```python
from build123d import *

# Parameters (mm, degrees)
SKETCH3_R           = 4.5
BOSS_EXTRUDE1_DEPTH = 18
FILLET1_R           = 5
FILLET2_R           = 5
CUT_EXTRUDE2_DEPTH  = 19.0000001


with BuildPart() as part:
    # Sketch3 → Boss-Extrude1 (new body)
    with BuildSketch(Plane.XY):
        with BuildLine():
            Line((-31.929873349, -122.5), (31.929873349, -122.5))
            ThreePointArc((31.929873349, -122.5), (38.210043039, -120.281996444), (41.704324989, -114.611893732))
            Line((41.704324989, -114.611893732), (73.308387301, 31.660797012))
            ThreePointArc((73.308387301, 31.660797012), (0, 122.5), (-73.308387301, 31.660797012))
            Line((-73.308387301, 31.660797012), (-41.704324989, -114.611893732))
            ThreePointArc((-41.704324989, -114.611893732), (-38.210043039, -120.281996444), (-31.929873349, -122.5))
        make_face()
        with Locations((50, -12.5)):
            Circle(SKETCH3_R, mode=Mode.SUBTRACT)
        with Locations((50, 87.5)):
            Circle(SKETCH3_R, mode=Mode.SUBTRACT)
        with Locations((-50, 87.5)):
            Circle(SKETCH3_R, mode=Mode.SUBTRACT)
        with Locations((-50, -12.5)):
            Circle(SKETCH3_R, mode=Mode.SUBTRACT)
        with BuildLine():
            Line((-31.929873349, -112.5), (-51.284518999, -22.921132901))
            ThreePointArc((-51.284518999, -22.921132901), (-39.736825778, -10.282511582), (-55.472323677, -3.538768301))
            Line((-55.472323677, -3.538768301), (-63.533935661, 33.772690744))
            ThreePointArc((-63.533935661, 33.772690744), (-64.271528905, 57.204152316), (-56.648842383, 79.373322021))
            ThreePointArc((-56.648842383, 79.373322021), (-41.800877501, 80.940702001), (-43.531035666, 95.770580418))
            ThreePointArc((-43.531035666, 95.770580418), (0, 112.5), (43.531035666, 95.770580418))
            ThreePointArc((43.531035666, 95.770580418), (41.800877501, 80.940702001), (56.648842383, 79.373322021))
            ThreePointArc((56.648842383, 79.373322021), (64.271528905, 57.204152316), (63.533935661, 33.772690744))
            Line((63.533935661, 33.772690744), (55.472323677, -3.538768301))
            ThreePointArc((55.472323677, -3.538768301), (39.736825778, -10.282511582), (51.284518999, -22.921132901))
            Line((51.284518999, -22.921132901), (31.929873349, -112.5))
            Line((31.929873349, -112.5), (-31.929873349, -112.5))
        make_face(mode=Mode.SUBTRACT)
    extrude(amount=BOSS_EXTRUDE1_DEPTH)

    # Fillet1
    fillet1_edges = [part.edges().sort_by_distance(p)[0] for p in [
        (-31.929873349, -112.5, 9),
        (31.929873349, -112.5, 9),
    ]]
    fillet(fillet1_edges, radius=FILLET1_R)

    # Fillet2
    fillet2_edges = [part.edges().sort_by_distance(p)[0] for p in [
        (51.284518999, -22.921132901, 9),
        (55.472323677, -3.538768301, 9),
        (56.648842383, 79.373322021, 9),
        (43.531035666, 95.770580418, 9),
        (-43.531035666, 95.770580418, 9),
        (-56.648842383, 79.373322021, 9),
        (-55.472323677, -3.538768301, 9),
        (-51.284518999, -22.921132901, 9),
    ]]
    fillet(fillet2_edges, radius=FILLET2_R)

    # Sketch5 → Cut-Extrude2 (cut, through all)
    with BuildSketch(Plane.XY.offset(18)):
        Polygon((47.724403212, -39.39837277), (54.444339069, -31.972010438), (57.506356145, -41.47554836), (172.58444794, 157.130363262), (-148.336678287, 157.130363262), (-57.506356145, -41.47554836), (-54.443982463, -31.973660914), (-47.723687693, -39.401684395), align=None)
    extrude(amount=-CUT_EXTRUDE2_DEPTH, mode=Mode.SUBTRACT)


solid = part.part
```
The listing builds one solid part. Answer for the finished solid, in the listing's coordinates (mm). A direction names the side the tool comes from. Give positions to 0.01 mm unless a question says otherwise; leave off trailing zeros. Order: outer loops, then holes, each group sorted by start corner. A loop starts at its lowest first (then second) coordinate and runs counter-clockwise, first axis right, second up.
1) Find section D-D on y = -116.5. Write down the section's boundary in (x, z).
Reported:
outline: (-41.1, 0) - (41.1, 0) - (41.1, 18) - (-41.1, 18) - close
2) For faces 4 (the face through (40.36, -73.49, 8.87)), 5 (the face through (-38.284, -120.222, 8.874)), determine the directions among +Z, -Z, +X, -X, +Y, -Y from which every point of the face is accessible in a straight line to the end or side of a thin tool.
Reported:
face 4: +Z, -Z, +Y
face 5: +Z, -Z, -X, -Y
3) Consider line 1 along Y through (x, z) = (19, 17); line 2 along X through (y, z) = (-50, 16.75); line 3 along X through (y, z) = (-42, 8). Determine where each line is inside the solid, lowest interval first.
Reported:
line 1: y = -122.5 to -112.5
line 2: x = -55.66 to -45.43, 45.43 to 55.66
line 3: x = -57.39 to -47.16, 47.16 to 57.39
4) Find section C-C on x = 1. Write down the section's boundary in (y, z), then the cut area to 3 significant figures.
Reported:
outline: (-122.5, 0) - (-112.5, 0) - (-112.5, 18) - (-122.5, 18) - close
area: 180 mm2
5) Find section B-B on y = -51. Write down the section's boundary in (x, z).
Reported:
outline: (-55.45, 0) - (-45.22, 0) - (-45.22, 18) - (-55.45, 18) - close; (45.22, 0) - (55.45, 0) - (55.45, 18) - (45.22, 18) - close
6) Given P1, Ø4, axis at x = -19, z = 9.5, coming from the +Y side; P2, Ø1, axis at y = -113, z = 13, coming from the -X side; P3, Ø3, axis at y = -54.5, z = 3.5, coming from the -X side, each flat-ended and moving along its own axis, determine where each tip first touches the part or whether it passes through.
Reported:
P1: stops at y = -112.5
P2: stops at x = -42.16
P3: stops at x = -55.02
7) Find section A-A on z = 11.5. Write down the section's boundary in (x, y).
Reported:
outline: (-57.51, -41.48) - (-41.7, -114.61) arc R10 ccw to (-31.93, -122.5) - (31.93, -122.5) arc R10 ccw to (41.7, -114.61) - (57.51, -41.48) - (54.44, -31.97) - (47.72, -39.4) - (32.78, -108.56) arc R5 cw to (27.89, -112.5) - (-27.89, -112.5) arc R5 cw to (-32.78, -108.56) - (-47.72, -39.4) - (-54.44, -31.97) - close
8) Determine the mould class of faces 1 (the face through (55.954, -36.657, 9.126)), 2 (the face through (51.037, -35.737, 9.126)), 3 (the face through (0, -114, 18)) for opening direction X: pulls with the +X half, pulls with the -X half, needs draft (parallel to the pull), parting line crosses it, or undercut.
Reported:
face 1: pulls with the +X half
face 2: undercut
face 3: needs draft
